Part print with two shaded views. Sizes in mm from the minimum x, y, z corner. Round coordinates to 2 decimals unless told otherwise and drop trailing zeros. Order: outer loops, then holes, each group sorted by start corner. A loop starts at its lowest first (then second) coordinate and runs counter-clockwise, first axis right, second up. Notation, with made-up numbers: M 55.25,15 L 96.25,15 A18 ccw 96.25,19 Z; hole C 41.5,13.25 d8. An arc over 180 degrees is marked long. Put each result on its own line as item: value.
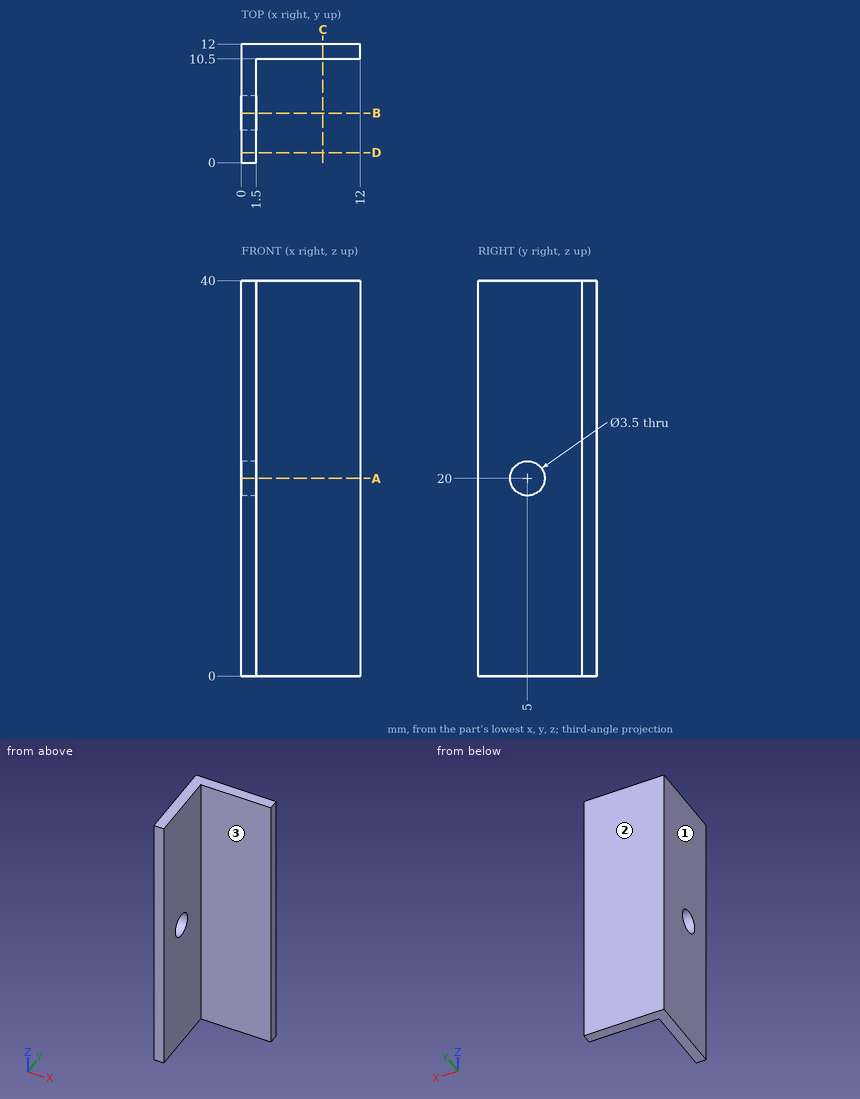
Item 1: Band-saw the part on C-C on x = 8.25. Give the cut face in (y, z), and give its area (3 significant figures).
Answers below:
outline: M 10.5,0 L 12,0 L 12,40 L 10.5,40 Z
area: 60.0 mm²
Item 2: Probe line 1 along Y through (x, z) = (0.5, 20); line 2 along Z through (x, y) = (0.55, 5); line 3 along X through (y, z) = (1, 15). List the from-to ranges inside material, lowest first. Write a range as [from, to].
Answers below:
line 1: [0, 3.25], [6.75, 12]
line 2: [0, 18.25], [21.75, 40]
line 3: [0, 1.5]
Item 3: Mould opens along Y. For the marked faces 1, 2 and 3 say: pulls with the +Y half, pulls with the -Y half, needs draft (parallel to the pull), parting line crosses it, or undercut.
Answers below:
face 1: needs draft
face 2: pulls with the +Y half
face 3: pulls with the -Y half
Item 4: Pin check, flat tips, straight feed: P1, Ø4.5, axis at y = 5, z = 20, coming from the -X side; P2, Ø3, axis at y = 6.5, z = 23, coming from the +X side; P3, Ø5, axis at x = 9, z = 23, coming from the -Y side. Stop position of each tip, or through.
Answers below:
P1: x = 0
P2: x = 1.5
P3: y = 10.5
Item 5: Band-saw the part on B-B on y = 5. Give the cut face in (x, z), and give its area (4 significant figures).
Answers below:
outline: M 0,0 L 1.5,0 L 1.5,18.25 L 0,18.25 Z; M 0,21.75 L 1.5,21.75 L 1.5,40 L 0,40 Z
area: 54.75 mm²
Item 6: Band-saw the part on A-A on z = 20. Give the cut face in (x, y).
Answers below:
outline: M 0,0 L 1.5,0 L 1.5,3.25 L 0,3.25 Z; M 0,6.75 L 1.5,6.75 L 1.5,10.5 L 12,10.5 L 12,12 L 0,12 Z
Item 7: Band-saw the part on D-D on y = 1. Give the cut face in (x, z).
Answers below:
outline: M 0,0 L 1.5,0 L 1.5,40 L 0,40 Z
